Part model, mm, in its own coordinate system. A direction names the side the tool comes from. Round coordinates to 2 decimals unless told otherwise and drop trailing zeros. Loops run counter-clockwise (first coordinate to the right, second up) from the corner with the lowest first, then second, coordinate; pieces in that order, holes last.
1) Band-saw the part on A-A, the plane x = 728.5. Write the cut outline in (y, z).
2) Probe line 1 (Y direction, x = 969, z = -17); line 2 (X direction, y = -17, z = 4); line 3 (X direction, y = -26, z = -7). List the from-to ranges inside material, lowest first.
3) Drop flat-ended pins along their axis: P1, Ø12, axis at x = 814.5, y = 16.5, coming from the -Z side (3 decimals); P2, Ø10.5, axis at x = 10, y = 23, coming from the -Z side; P3, Ø12, axis at x = 770, y = 9.5, coming from the +Z side; P4, Ø12, axis at x = 732.5, y = -11.5, coming from the -Z side. Give the stop position or say it passes through.
4) Band-saw the part on B-B, the plane x = 1010. Write the cut outline in (y, z).
5) 3-axis set-ups, long thin cutter, end or side, ignore diameter. For faces 4 (the flat face through (20, 7, -8)), 5 (the flat face through (965, -30, -9)), 6 (the flat face through (1087, 0, -30)), 7 (the flat face through (1087, 30, 0)): which of +Z, -Z, +X, -X, +Y, -Y reach the whole face in a straight line?
6) Mould opens along Z. For faces 1 (the cylindrical face through (1006.622, 11.923, 3.755)), 2 (the flat face through (1070, 0, -35.58)), 3 (the flat face through (965, 30, -9)) say: +Z half, -Z half, draft (parallel to the pull), parting line (faces both ways), or undercut.
from build123d import *

# Parameters (mm, degrees)
F0_R      = 8
F1_DEPTH  = 980
F3_DEPTH  = 30
F5_DEPTH  = 20
F6_R      = 12.5
F7_DEPTH  = 57
F8_R      = 3.3
F9_DEPTH  = 43.001
F10_W     = 60
F10_H     = 60
F11_DEPTH = 101
F13_DEPTH = 32.5


# Not quite as in the source:
# - a feature names something its author has since deleted; it is built from what else it names


with BuildPart() as f1:
    # F0 (on Right) → F1 (new body)
    with BuildSketch(Plane.YZ):
        Circle(F0_R)
    extrude(amount=F1_DEPTH)

    # F2 (on face) → F3 (join)
    with BuildSketch(Plane.YZ.offset(980)):
        Polygon((30, 7.5), (17, 7.5), (17, 18), (-17, 18), (-17, 7.5), (-30, 7.5), (-30, -25), (30, -25), align=None)
    extrude(amount=-F3_DEPTH)

    # F4 (on face) → F5 (join)
    with BuildSketch(Plane(origin=(0, 0, 0), x_dir=(0, -1, 0), z_dir=(-1, 0, 0))):
        Polygon((17, 7.5), (17, 18), (-17, 18), (-17, 7.5), (-30, 7.5), (-30, -25), (30, -25), (30, 7.5), align=None)
    extrude(amount=-F5_DEPTH)

    # F6 (on face) → F7 (join)
    with BuildSketch(Plane.YZ.offset(980)):
        Circle(F6_R)
    extrude(amount=F7_DEPTH)

    # F8 (on face) → F9 (cut, through all)
    with BuildSketch(Plane.XY.offset(18)):
        with Locations((956, 23)):
            Circle(F8_R)
        with Locations((969, 23)):
            Circle(F8_R)
        with Locations((956, -23)):
            Circle(F8_R)
        with Locations((969, -23)):
            Circle(F8_R)
        with Locations((10, 23)):
            Circle(F8_R)
        with Locations((10, -23)):
            Circle(F8_R)
    extrude(amount=-F9_DEPTH, mode=Mode.SUBTRACT)

    # F10 (on face) → F11 (join)
    with BuildSketch(Plane.YZ.offset(1037)):
        Rectangle(F10_W, F10_H)
    extrude(amount=F11_DEPTH)

    # F12 (on Front) → F13 (join, symmetric)
    with BuildSketch(Plane.XZ):
        Polygon((1037, 30), (1034, 30), (1034, -38.58), (1102.58, -38.58), (1102.58, -35.58), (1037, -35.58), align=None)
    extrude(amount=F13_DEPTH, both=True)


solid = f1.part
Reported:
1. outline: circle Ø16 at (0, 0)
2. line 1: y = -30 to -26.3, -19.7 to 19.7, 26.3 to 30
2. line 2: x = 0 to 20, 950 to 980, 1034 to 1138
2. line 3: x = 0 to 8.63, 11.37 to 20, 950 to 954.63, 957.37 to 967.63, 970.37 to 980, 1034 to 1138
3. P1: passes through
3. P2: stops at z = -25
3. P3: stops at z = 7.19
3. P4: stops at z = -5.81
4. outline: circle Ø25 at (0, 0)
5. face 4: none
5. face 5: +Z, -Z, -X, -Y
5. face 6: +X, +Y, -Y
5. face 7: +Z, +X, +Y
6. face 1: parting line
6. face 2: undercut
6. face 3: draft
